```python
from build123d import *

# Parameters (mm, degrees)
SALIENTE_EXTRUIR1_DEPTH = 11
SALIENTE_EXTRUIR2_DEPTH = 0.5
SALIENTE_EXTRUIR3_DEPTH = 1.5
SALIENTE_EXTRUIR3_TAPER = 45
CORTAR_EXTRUIR1_DEPTH   = 6
CROQUIS7_W              = 6.69
CROQUIS7_H              = 1.2
SALIENTE_EXTRUIR4_DEPTH = 4.7
REDONDEO1_R             = 0.1
SALIENTE_EXTRUIR5_DEPTH = 1.5


with BuildPart() as part:
    # Croquis1 → Saliente-Extruir1 (new body)
    with BuildSketch(Plane(origin=(0, 0, 0), x_dir=(1, 0, 0), z_dir=(0, 1, 0))):
        with BuildLine():
            Line((-5.6, -2.6), (5.6, -2.6))
            ThreePointArc((5.6, -2.6), (5.953553391, -2.453553391), (6.1, -2.1))
            Line((6.1, -2.1), (6.1, 2.1))
            ThreePointArc((6.1, 2.1), (5.953553391, 2.453553391), (5.6, 2.6))
            Line((5.6, 2.6), (-5.6, 2.6))
            ThreePointArc((-5.6, 2.6), (-5.953553391, 2.453553391), (-6.1, 2.1))
            Line((-6.1, 2.1), (-6.1, -2.1))
            ThreePointArc((-6.1, -2.1), (-5.953553391, -2.453553391), (-5.6, -2.6))
        make_face()
    extrude(amount=-SALIENTE_EXTRUIR1_DEPTH)

    # Croquis2 → Saliente-Extruir2 (add)
    with BuildSketch(Plane(origin=(0, 0, 0), x_dir=(1, 0, 0), z_dir=(0, 1, 0))):
        with BuildLine():
            Line((-3.8, -4.1), (3.8, -4.1))
            ThreePointArc((3.8, -4.1), (7.9, 0), (3.8, 4.1))
            Line((3.8, 4.1), (-3.8, 4.1))
            ThreePointArc((-3.8, 4.1), (-7.9, 0), (-3.8, -4.1))
        make_face()
    extrude(amount=SALIENTE_EXTRUIR2_DEPTH)

    # Croquis3 → Saliente-Extruir3 (add)
    with BuildSketch(Plane(origin=(0, 0.5, 0), x_dir=(1, 0, 0), z_dir=(0, 1, 0))):
        with BuildLine():
            Line((-3.8, -4.1), (3.8, -4.1))
            ThreePointArc((3.8, -4.1), (7.9, 0), (3.8, 4.1))
            Line((3.8, 4.1), (-3.8, 4.1))
            ThreePointArc((-3.8, 4.1), (-7.9, 0), (-3.8, -4.1))
        make_face()
    extrude(amount=SALIENTE_EXTRUIR3_DEPTH, taper=SALIENTE_EXTRUIR3_TAPER)

    # Croquis6 → Cortar-Extruir1 (cut)
    with BuildSketch(Plane(origin=(0, 2, 0), x_dir=(1, 0, 0), z_dir=(0, 1, 0))):
        with BuildLine():
            Line((-3.27, 1.28), (3.27, 1.28))
            ThreePointArc((3.27, 1.28), (3.977106781, 0.987106781), (4.27, 0.28))
            Line((4.27, 0.28), (4.27, -0.28))
            ThreePointArc((4.27, -0.28), (3.977106781, -0.987106781), (3.27, -1.28))
            Line((3.27, -1.28), (-3.27, -1.28))
            ThreePointArc((-3.27, -1.28), (-3.977106781, -0.987106781), (-4.27, -0.28))
            Line((-4.27, -0.28), (-4.27, 0.28))
            ThreePointArc((-4.27, 0.28), (-3.977106781, 0.987106781), (-3.27, 1.28))
        make_face()
    extrude(amount=-CORTAR_EXTRUIR1_DEPTH, mode=Mode.SUBTRACT)

    # Croquis7 → Saliente-Extruir4 (add)
    with BuildSketch(Plane(origin=(0, -4, 0), x_dir=(1, 0, 0), z_dir=(0, 1, 0))):
        Rectangle(CROQUIS7_W, CROQUIS7_H)
    extrude(amount=SALIENTE_EXTRUIR4_DEPTH)

    # Redondeo1
    redondeo1_edges = [part.edges().sort_by_distance(p)[0] for p in [
        (3.345, -1.65, 0.6),
        (3.345, -1.65, -0.6),
        (-3.345, -1.65, -0.6),
        (-3.345, -1.65, 0.6),
    ]]
    fillet(redondeo1_edges, radius=REDONDEO1_R)

    # Croquis8 → Saliente-Extruir5 (add, symmetric)
    with BuildSketch(Plane.XY):
        Polygon((-6.1, 0), (-7.9, -3), (-6.1, -11), (-6.1, -8.722222222), (-7.368246767, -3.085569927), (-6.1, -0.971825316), align=None)
        Polygon((6.1, -0.971825316), (6.1, 0), (7.9, -3), (6.1, -11), (6.1, -8.722222222), (7.368246767, -3.085569927), align=None)
    extrude(amount=SALIENTE_EXTRUIR5_DEPTH, both=True)


solid = part.part
```
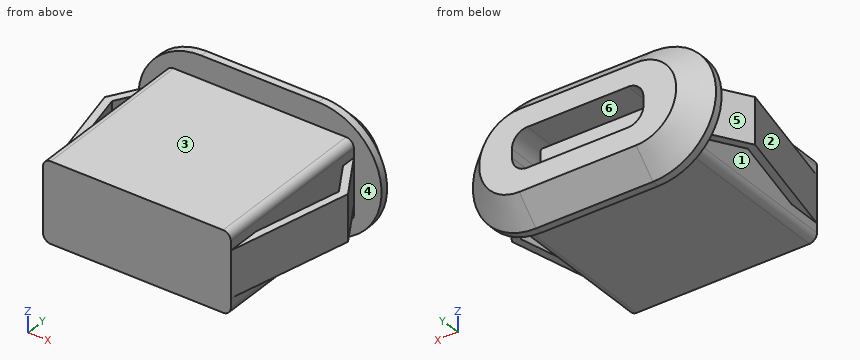
Input: part model. Units: mm. Frame: model coordinates. Face numbers are marked on the shaded views. A direction names the side the tool comes from. Coordinates: 2 decimals unless noted, no trailing zeros. Loops run counter-clockwise (first coordinate to the right, second up) from the corner with the lowest first, then second, coordinate; pieces in that order, holes last.
Q1. Set-up query: the marked faces 4, 5 and 6. Return all of +Z, -Z, +X, -X, +Y, -Y with unobstructed straight access to the full face (end or side cutting, diameter ignored); none if empty.
Results are:
face 4: none
face 5: +Z, -Z, -X
face 6: +Y
Q2. Line query: line 1 along Z through (x, y) = (2.25, -1.5); line 2 along X through (y, z) = (-4.5, 0.5); line 3 along X through (y, z) = (-7.5, 0.5) (1 decimal). Output: solid intervals per line, ascending.
Results are:
line 1: z = -2.6 to -1.28, -0.6 to 0.6, 1.28 to 2.6
line 2: x = -7.56 to -7.05, -6.1 to 6.1, 7.05 to 7.56
line 3: x = -6.9 to -6.4, -6.1 to 6.1, 6.4 to 6.9
Q3. Section A-A, the plane z = 0. Return the cut outline in (x, y) (3 decimals).
Results are:
outline: (-7.9, -3) - (-6.1, -11) - (6.1, -11) - (7.9, -3) - (6.1, 0) - (7.9, 0) - (7.9, 0.5) - (6.4, 2) - (4.27, 2) - (4.27, -4) - (3.345, -4) - (3.345, 0.7) - (-3.345, 0.7) - (-3.345, -4) - (-4.27, -4) - (-4.27, 2) - (-6.4, 2) - (-7.9, 0.5) - (-7.9, 0) - (-6.1, 0) - close; hole (-7.368, -3.086) - (-6.1, -8.722) - (-6.1, -0.972) - close; hole (6.1, -8.722) - (7.368, -3.086) - (6.1, -0.972) - close
Q4. Section B-B, the plane y = -7.5. Return the cut outline in (x, z) (1 decimal).
Results are:
outline: (-6.9, -1.5) - (-6.4, -1.5) - (-6.4, 1.5) - (-6.9, 1.5) - close; (-6.1, -2.1) arc R0.5 ccw to (-5.6, -2.6) - (5.6, -2.6) arc R0.5 ccw to (6.1, -2.1) - (6.1, 2.1) arc R0.5 ccw to (5.6, 2.6) - (-5.6, 2.6) arc R0.5 ccw to (-6.1, 2.1) - close; (6.4, -1.5) - (6.9, -1.5) - (6.9, 1.5) - (6.4, 1.5) - close
Q5. Contact query for flat-ended pins moving along their axis: pin 1 (5 mm diameter, centred on x = -1, y = -2, fed in from +Z); pin 2 (1.5 mm diameter, centred on x = -3, y = -3.5, fed in from +Z); pin 3 (1 mm diameter, centred on x = 1, z = 0, fed in from +Y); pin 4 (4.5 mm diameter, centred on y = -7, z = 0.5, fed in from -X). Output: stop coordinate, or through.
Results are:
pin 1: stops at z = 4.1
pin 2: stops at z = 2.6
pin 3: stops at y = 0.7
pin 4: stops at x = -7.51
Q6. Section C-C, the plane x = -1.75. Return the cut outline in (y, z), and give its area (3 significant figures).
Results are:
outline: (-11, -2.6) - (0, -2.6) - (0, -4.1) - (0.5, -4.1) - (2, -2.6) - (2, -1.28) - (-4, -1.28) - (-4, -0.6) - (0.7, -0.6) - (0.7, 0.6) - (-4, 0.6) - (-4, 1.28) - (2, 1.28) - (2, 2.6) - (0.5, 4.1) - (0, 4.1) - (0, 2.6) - (-11, 2.6) - close
area: 61.6 mm2
Q7. Mould query, pull axis Y, two halves, no side actions, for the marked faces 1, 2 and 3. Classes: +Y half, -Y half, draft (parallel to the pull), parting line (faces both ways), or undercut.
Results are:
face 1: undercut
face 2: -Y half
face 3: draft
